from build123d import *

# Parameters (mm, degrees)
BOSS_EXTRUDE1_DEPTH = 19
SKETCH2_W           = 4.5
SKETCH2_H           = 4.5
BOSS_EXTRUDE2_DEPTH = 19
FILLET1_R           = 10
FILLET2_R           = 10
FILLET3_R           = 1
SKETCH3_R           = 1.5
CUT_EXTRUDE1_DEPTH  = 19
SKETCH4_W           = 32
SKETCH4_H           = 3
CUT_EXTRUDE2_DEPTH  = 47.238512087
SKETCH5_W           = 32
SKETCH5_H           = 39
SKETCH5_R           = 1.5
BOSS_EXTRUDE3_DEPTH = 3
SKETCH6_R           = 7.5
CUT_EXTRUDE3_DEPTH  = 33.984845005


with BuildPart() as part:
    # Sketch1 → Boss-Extrude1 (new body)
    with BuildSketch(Plane.XY):
        with BuildLine():
            Line((-16, 24), (-16, 0))
            ThreePointArc((-16, 0), (-15.491933385, 4), (-14, 7.745966692))
            Line((-14, 7.745966692), (-14, 22))
            Line((-14, 22), (-14, 24))
            Line((-14, 24), (-16, 24))
        make_face()
        with BuildLine():
            ThreePointArc((-14, 7.745966692), (-15.491933385, 4), (-16, 0))
            ThreePointArc((-16, 0), (-15.491933385, -4), (-14, -7.745966692))
            Line((-14, -7.745966692), (-14, 0))
            Line((-14, 0), (-14, 7.745966692))
        make_face()
        with BuildLine():
            ThreePointArc((-14, -7.745966692), (-15.491933385, -4), (-16, 0))
            Line((-16, 0), (-16, -15))
            Line((-16, -15), (-5.567764363, -15))
            ThreePointArc((-5.567764363, -15), (-7.514407784, -14.125638947), (-9.327379053, -13))
            Line((-9.327379053, -13), (-14, -13))
            Line((-14, -13), (-14, -7.745966692))
        make_face()
        with BuildLine():
            ThreePointArc((-9.327379053, -13), (-7.514407784, -14.125638947), (-5.567764363, -15))
            Line((-5.567764363, -15), (5.567764363, -15))
            ThreePointArc((5.567764363, -15), (7.514407784, -14.125638947), (9.327379053, -13))
            Line((9.327379053, -13), (5.196152423, -13))
            ThreePointArc((5.196152423, -13), (0, -14), (-5.196152423, -13))
            Line((-5.196152423, -13), (-9.327379053, -13))
        make_face()
        with BuildLine():
            Line((5.196152423, -13), (-5.196152423, -13))
            ThreePointArc((-5.196152423, -13), (0, -14), (5.196152423, -13))
        make_face()
        with BuildLine():
            ThreePointArc((9.327379053, -13), (7.514407784, -14.125638947), (5.567764363, -15))
            Line((5.567764363, -15), (16, -15))
            Line((16, -15), (16, 0))
            ThreePointArc((16, 0), (15.491933385, -4), (14, -7.745966692))
            Line((14, -7.745966692), (14, -13))
            Line((14, -13), (9.327379053, -13))
        make_face()
        with BuildLine():
            ThreePointArc((16, 0), (15.491933385, 4), (14, 7.745966692))
            Line((14, 7.745966692), (14, 0))
            Line((14, 0), (14, -7.745966692))
            ThreePointArc((14, -7.745966692), (15.491933385, -4), (16, 0))
        make_face()
        with BuildLine():
            Line((14, 22), (14, 7.745966692))
            ThreePointArc((14, 7.745966692), (15.491933385, 4), (16, 0))
            Line((16, 0), (16, 24))
            Line((16, 24), (14, 24))
            Line((14, 24), (14, 22))
        make_face()
    extrude(amount=BOSS_EXTRUDE1_DEPTH)

    # Sketch2 → Boss-Extrude2 (add)
    with BuildSketch(Plane.XY.offset(19)):
        with Locations((-11.75, 21.75)):
            Rectangle(SKETCH2_W, SKETCH2_H)
        with Locations((11.75, 21.75)):
            Rectangle(SKETCH2_W, SKETCH2_H)
    extrude(amount=-BOSS_EXTRUDE2_DEPTH)

    # Fillet1
    fillet1_edges = [part.edges().sort_by_distance(p)[0] for p in [
        (-14, -13, 9.5),
    ]]
    fillet(fillet1_edges, radius=FILLET1_R)

    # Fillet2
    fillet2_edges = [part.edges().sort_by_distance(p)[0] for p in [
        (14, -13, 9.5),
    ]]
    fillet(fillet2_edges, radius=FILLET2_R)

    # Fillet3
    fillet3_edges = [part.edges().sort_by_distance(p)[0] for p in [
        (-14, 19.5, 9.5),
        (14, 19.5, 9.5),
    ]]
    fillet(fillet3_edges, radius=FILLET3_R)

    # Sketch3 → Cut-Extrude1 (cut)
    with BuildSketch(Plane.XY.offset(19)):
        with Locations((-12.5, 21.75)):
            Circle(SKETCH3_R)
        with Locations((-13, -12)):
            Circle(SKETCH3_R)
        with Locations(Location((12.5, 21.75, 0), (0, 0, 180))):
            Circle(SKETCH3_R)
        with Locations(Location((13, -12, 0), (0, 0, 180))):
            Circle(SKETCH3_R)
    extrude(amount=-CUT_EXTRUDE1_DEPTH, mode=Mode.SUBTRACT)

    # Sketch4 → Cut-Extrude2 (cut, through all)
    with BuildSketch(Plane(origin=(0, 24, 0), x_dir=(1, 0, 0), z_dir=(0, 1, 0))):
        with Locations((0, -17.5)):
            Rectangle(SKETCH4_W, SKETCH4_H)
    extrude(amount=-CUT_EXTRUDE2_DEPTH, mode=Mode.SUBTRACT)

    # Sketch5 → Boss-Extrude3 (add)
    with BuildSketch(Plane.XY.offset(16)):
        with Locations((0, 4.5)):
            Rectangle(SKETCH5_W, SKETCH5_H)
        with Locations((-12.5, 21.75)):
            Circle(SKETCH5_R, mode=Mode.SUBTRACT)
        with Locations(Location((12.5, 21.75, 0), (0, 0, 180))):
            Circle(SKETCH5_R, mode=Mode.SUBTRACT)
        with Locations((-13, -12)):
            Circle(SKETCH5_R, mode=Mode.SUBTRACT)
        with Locations(Location((13, -12, 0), (0, 0, 180))):
            Circle(SKETCH5_R, mode=Mode.SUBTRACT)
    extrude(amount=-BOSS_EXTRUDE3_DEPTH)

    # Sketch6 → Cut-Extrude3 (cut, through all)
    with BuildSketch(Plane.XY.offset(16)):
        Circle(SKETCH6_R)
    extrude(amount=-CUT_EXTRUDE3_DEPTH, mode=Mode.SUBTRACT)


solid = part.part
Geometry: final body of the model. Coordinates: model frame, mm. A direction names the side the tool comes from. Give positions to 0.01 mm unless a question says otherwise; leave off trailing zeros. Order: outer loops, then holes, each group sorted by start corner. A loop starts at its lowest first (then second) coordinate and runs counter-clockwise, first axis right, second up. Notation, with made-up numbers: (-39, 55) -> (17, 55) arc R16 ccw to (17, 85) -> close; hole circle Ø9 at (15, 33). An arc over 180 degrees is marked (long way). Put each result on its own line as item: value.
Q1. Pin query (flat end, axial travel): pin 1 (5 mm diameter, centred on x = 4.5, y = -11, fed in from -Z); pin 2 (1 mm diameter, centred on x = -5.5, y = 8.5, fed in from -Z); pin 3 (4 mm diameter, centred on x = -1, z = 6, fed in from +Y); pin 4 (3 mm diameter, centred on x = -7.5, z = 8, fed in from +Y). Return the tip coordinate at first contact, or that it passes through.
Here are the results:
pin 1: stops at z = 0
pin 2: stops at z = 13
pin 3: stops at y = -13
pin 4: stops at y = -11.66
Q2. Section A-A, the plane y = 0. Return loops of the section in (x, z).
Here are the results:
outline: (-16, 0) -> (-14, 0) -> (-14, 13) -> (-7.5, 13) -> (-7.5, 16) -> (-16, 16) -> close; (7.5, 13) -> (14, 13) -> (14, 0) -> (16, 0) -> (16, 16) -> (7.5, 16) -> close
Q3. Section C-C, the plane z = 5.5. Return loops of the section in (x, y), then the cut area to 3 significant figures.
Here are the results:
outline: (-16, -15) -> (16, -15) -> (16, 24) -> (9.5, 24) -> (9.5, 19.5) -> (13, 19.5) arc R1 cw to (14, 18.5) -> (14, -3) arc R10 cw to (4, -13) -> (-4, -13) arc R10 cw to (-14, -3) -> (-14, 18.5) arc R1 cw to (-13, 19.5) -> (-9.5, 19.5) -> (-9.5, 24) -> (-16, 24) -> close; hole circle Ø3 at (-13, -12); hole circle Ø3 at (-12.5, 21.75); hole circle Ø3 at (12.5, 21.75); hole circle Ø3 at (13, -12)
area: 268 mm^2
Q4. Draft query along Y for faces 4 (the face through (11, 19.5, 7)), 5 (the face through (0, 9, 16)), 6 (the face through (-0.2, 24, 13.4)). Return one class per face: released by +Y, released by -Y, zero draft, split by the parting line, or undercut.
Here are the results:
face 4: undercut
face 5: zero draft
face 6: released by +Y
Q5. Section D-D, the plane x = 0. Return loops of the section in (y, z).
Here are the results:
outline: (-15, 0) -> (-13, 0) -> (-13, 13) -> (-7.5, 13) -> (-7.5, 16) -> (-15, 16) -> close; (7.5, 13) -> (24, 13) -> (24, 16) -> (7.5, 16) -> close
Q6. Material intervals for L1, parallel to X at y = 6, z = 3; L2, parallel to Y at x = -13, z = 6.25; L3, parallel to Y at x = -3, z = 4, sorted ascending.
Here are the results:
L1: x = -16 to -14, 14 to 16
L2: y = -15 to -13.5, -10.5 to -7.36, 19.5 to 20.34, 23.16 to 24
L3: y = -15 to -13
Q7. Section B-B, the plane y = 21.75. Return loops of the section in (x, z), then the cut area to 3 significant figures.
Here are the results:
outline: (-16, 0) -> (-14, 0) -> (-14, 16) -> (-16, 16) -> close; (-11, 0) -> (-9.5, 0) -> (-9.5, 13) -> (9.5, 13) -> (9.5, 0) -> (11, 0) -> (11, 16) -> (-11, 16) -> close; (14, 0) -> (16, 0) -> (16, 16) -> (14, 16) -> close
area: 169 mm^2
Q8. Reachability of faces 1 (the face through (12.695, 20.263, 8.112)), 2 (the face through (0, 10, 13)), 3 (the face through (9.5, 22, 7)) from +Z, -Z, +X, -X, +Y, -Y: full face, straight path, thin tool, end or side. Return the list, or none.
Here are the results:
face 1: +Z, -Z
face 2: -Z
face 3: -Z, +Y
